Read the model definition and answer for the solid it produces. Units are mm, in the model's axes. A direction names the side the tool comes from. Give positions to 0.01 mm unless a question says otherwise; leave off trailing zeros. Loops run counter-clockwise (first coordinate to the right, second up) from the corner with the lowest first, then second, coordinate; pieces in that order, holes last. Notation, with made-up numbers: (50.25, 25.25) -> (108.25, 25.25) arc R23 ccw to (108.25, 59.25) -> close; hole circle Ø7 at (-16.75, 39). An arc over 180 degrees is marked (long way). Write each question's results on one line, items separated by ' | '. Start each with the question number.
Item 1: Find the intervals of material crossed by line 1 (X direction, y = 0.15, z = 5.25); line 2 (Z direction, x = 4.5, y = -0.35); line 3 (Y direction, x = 8.25, z = 4.75), in increasing order.
Item 2: Section D-D on x = 0.25 is taken. Write down the section's boundary in (y, z).
Item 3: Each of these flat-tipped pins is pushed along its axis until it touches: P1, Ø1.5, axis at x = 9, y = -0.5, coming from the +Z side; P2, Ø1, axis at x = -0.5, y = 1, coming from the +Z side; P3, Ø1.6, axis at x = 12.5, y = 1, coming from the -Z side. Where does it stop, or does it pass through?
Item 4: Section A-A on y = 1.6 is taken. Write down the section's boundary in (x, z), and give its area (3 significant figures).
Item 5: Section C-C on z = 0.5 is taken. Write down the section's boundary in (x, y).
Item 6: Section B-B on x = 5.5 is taken. Write down the section's boundary in (y, z).
Item 7: Which of the six approach directions +Z, -Z, +X, -X, +Y, -Y give full straight-line access (tool end or side, diameter ignored) to faces 1 (the cylindrical face through (13, 0, 3.5)), 2 (the cylindrical face through (7.64, 0.02, 4.86)), 3 (the flat face through (-1.6, -1.6, 3)), 4 (the flat face through (-1.5, 1.6, 2.2))?
```python
from build123d import *

# Parameters (mm, degrees)
EXTRUDE_1_DEPTH = 4
EXTRUDE_START   = -2.2
SKETCH_2_W      = 15
SKETCH_2_H      = 4
EXTRUDE_2_DEPTH = 0.8
SKETCH_3_R      = 0.5
EXTRUDE_3_DEPTH = 1
FILLET_1_R      = 0.5
SKETCH_4_R      = 0.4
EXTRUDE_4_DEPTH = 1.75


with BuildPart() as part:
    # 草图1 → 凸台-拉伸1 (new body)
    with BuildSketch(Plane.XY):
        with BuildLine():
            Line((0, 2), (11, 2))
            ThreePointArc((11, 2), (13, 0), (11, -2))
            Line((11, -2), (0, -2))
            ThreePointArc((0, -2), (-2, 0), (0, 2))
        make_face()
    extrude(amount=EXTRUDE_1_DEPTH)

    # 草图2 → 凸台-拉伸2 (add)
    with BuildSketch(Plane(origin=(0, 0, 0), x_dir=(-1, 0, 0), z_dir=(0, 0, -1)).offset(EXTRUDE_START)):
        with Locations((-5.5, 0)):
            Rectangle(SKETCH_2_W, SKETCH_2_H)
    extrude(amount=-EXTRUDE_2_DEPTH)

    # 草图3 → 凸台-拉伸3 (add)
    with BuildSketch(Plane(origin=(0, 0, 0), x_dir=(-1, 0, 0), z_dir=(0, 0, -1))):
        with Locations(Location((-8.04, 0, 0), (0, 0, 180))):
            Circle(SKETCH_3_R)
        with Locations(Location((-5.5, 0, 0), (0, 0, 180))):
            Circle(SKETCH_3_R)
        with Locations(Location((-2.96, 0, 0), (0, 0, 180))):
            Circle(SKETCH_3_R)
    extrude(amount=EXTRUDE_3_DEPTH)

    # 圆角1
    fillet_1_edges = [part.edges().sort_by_distance(p)[0] for p in [
        (7.54, 0, -1),
        (5, 0, -1),
        (2.46, 0, -1),
    ]]
    fillet(fillet_1_edges, radius=FILLET_1_R)

    # 草图4 → 凸台-拉伸4 (add)
    with BuildSketch(Plane.XY.offset(4)):
        with Locations((2.96, 0)):
            Circle(SKETCH_4_R)
        with Locations((5.5, 0)):
            Circle(SKETCH_4_R)
        with Locations((8.04, 0)):
            Circle(SKETCH_4_R)
    extrude(amount=EXTRUDE_4_DEPTH)


solid = part.part
```
Findings:
1) line 1: 2.59 to 3.33, 5.13 to 5.87, 7.67 to 8.41 | line 2: 0 to 4 | line 3: -0.34 to 0.34
2) outline: (-2, 0) -> (2, 0) -> (2, 4) -> (-2, 4) -> close
3) P1: z = 5.75 | P2: z = 4 | P3: z = 0
4) outline: (-2, 2.2) -> (-1.2, 2.2) -> (-1.2, 0) -> (12.2, 0) -> (12.2, 2.2) -> (13, 2.2) -> (13, 3) -> (12.2, 3) -> (12.2, 4) -> (-1.2, 4) -> (-1.2, 3) -> (-2, 3) -> close | area: 54.9 mm2
5) outline: (0, -2) -> (11, -2) arc R2 ccw to (11, 2) -> (0, 2) arc R2 ccw to start
6) outline: (-2, 0) -> (-0.5, 0) -> (-0.5, -0.5) arc R0.5 ccw to (0.5, -0.5) -> (0.5, 0) -> (2, 0) -> (2, 4) -> (0.4, 4) -> (0.4, 5.75) -> (-0.4, 5.75) -> (-0.4, 4) -> (-2, 4) -> close
7) face 1: +Z, +X | face 2: +Z | face 3: +Z, -X, -Y | face 4: -Z, -X, +Y
